Design review of the part shown in the three views and the two pictorial views. Dimensions are in mm from the part's minimum x, y and z. Round coordinates to 2 decimals unless told otherwise and drop trailing zeros. Loops run counter-clockwise (first coordinate to the right, second up) from the corner with the lowest first, then second, coordinate; pieces in that order, holes last. Notation, with made-up numbers: (70, -27) -> (116, -27) arc R24 cw to (116, -3) -> close; hole circle Ø1 at (16, 59.25). An arc over 180 degrees is marked (long way). Use a Markdown table: item, result. Add a question column.
1) Consider section A-A on z = 36. Give the boundary of the cut face in (x, y), plus the area to 3 significant figures.
2) Insertion check: pin 1 (11 mm diameter, centred on x = 409, z = 36, fed in from +Y); pin 2 (3 mm diameter, centred on y = 4.5, z = 98.5, fed in from +X); pin 3 (4 mm diameter, centred on x = 682, y = 3, fed in from -Z); pin 4 (2.5 mm diameter, centred on y = 3.5, z = 206, fed in from -X). Each pin has a flat end and moves straight along its axis. Give the tip position at first contact, or say it passes through.
3) Wall thickness on probe 1 along X at (y, z) = (2, 214); probe 2 along Z at (x, y) = (409, 6); probe 3 along X at (y, z) = (6.25, 41.5): over which ranges is each line inside the solid? List them lowest first.
4) Consider section C-C on y = 3.25. State how many separate pieces and enclosed holes the cut face has, plus the area to 3 significant figures.
5) Consider section D-D on z = 102.5. Give the boundary of the cut face in (x, y).
6) Consider section B-B on x = 193. Give the boundary of the cut face in (y, z), plus the area to 3 significant figures.
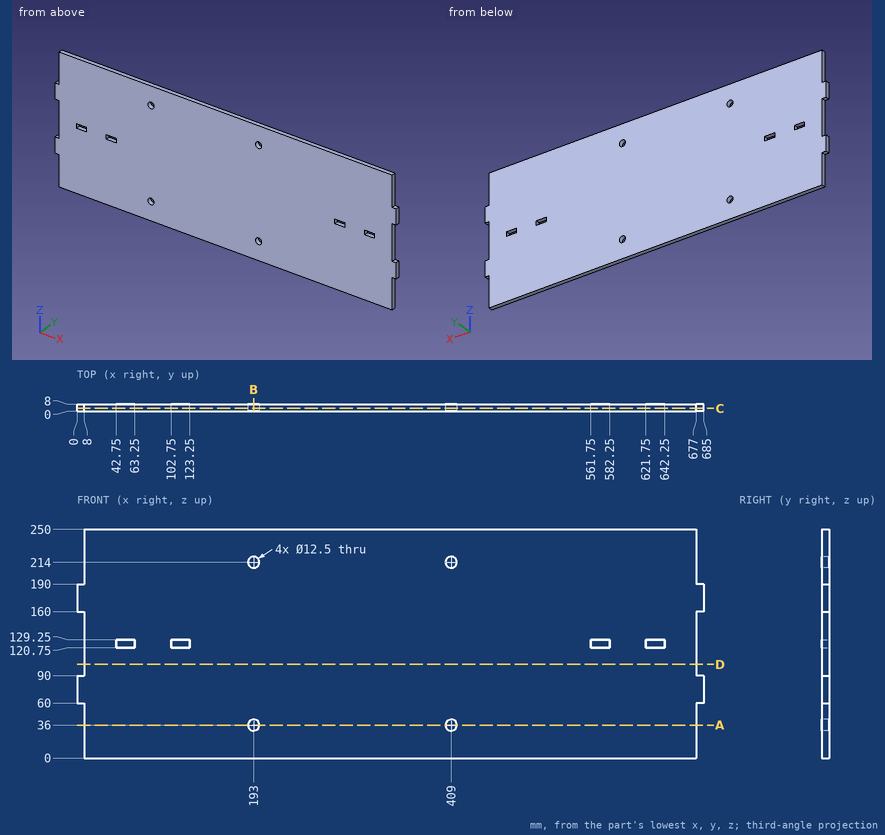
Result set:
| question | item | result |
|---|---|---|
| 1 | outline | (8, 0) -> (186.75, 0) -> (186.75, 8) -> (8, 8) -> close; (199.25, 0) -> (402.75, 0) -> (402.75, 8) -> (199.25, 8) -> close; (415.25, 0) -> (677, 0) -> (677, 8) -> (415.25, 8) -> close |
| 1 | area | 5,150 mm2 |
| 2 | pin 1 | through |
| 2 | pin 2 | x = 677 |
| 2 | pin 3 | z = 60 |
| 2 | pin 4 | x = 8 |
| 3 | probe 1 | 8 to 186.75, 199.25 to 402.75, 415.25 to 677 |
| 3 | probe 2 | 0 to 29.75, 42.25 to 207.75, 220.25 to 250 |
| 3 | probe 3 | 8 to 190.03, 195.97 to 406.03, 411.97 to 677 |
| 4 | separate pieces | 1 |
| 4 | enclosed holes | 8 |
| 4 | area | 167,000 mm2 |
| 5 | outline | (8, 0) -> (677, 0) -> (677, 8) -> (8, 8) -> close |
| 6 | outline | (0, 0) -> (8, 0) -> (8, 29.75) -> (0, 29.75) -> close; (0, 42.25) -> (8, 42.25) -> (8, 207.75) -> (0, 207.75) -> close; (0, 220.25) -> (8, 220.25) -> (8, 250) -> (0, 250) -> close |
| 6 | area | 1,800 mm2 |
